Build history of the part. All positions in model axes, mm. A direction names the side the tool comes from. Round coordinates to 2 decimals unless told otherwise and drop trailing zeros. Order: outer loops, then holes, each group sorted by start corner. A loop starts at its lowest first (then second) coordinate and runs counter-clockwise, first axis right, second up. Notation, with made-up numbers: M -32.5,12.5 L -19.5,12.5 A31 cw -19.5,46.5 Z; hole C -13,67.5 d4. An arc over 180 degrees is marked long. One line per item, written item: value. Start each with the question number.
Item 1: Band-saw the part on A-A, the plane z = 0. Write the cut outline in (x, y).
Item 2: Tool access for faces 4 (the flat face through (5, 5, -7)), 5 (the flat face through (-5, 0, -6)): list every direction of +Z, -Z, +X, -X, +Y, -Y with a clear straight run to the whole face (end or side of a thin tool).
Item 3: Two-plate mould, pull along Z, no slides. Class faces 1 (the flat face through (22.5, 3, 0)), 2 (the cylindrical face through (-21.61, 3.04, 4.13)), 3 (the cylindrical face through (-1.139, 2.218, 7.514)): +Z half, -Z half, draft (parallel to the pull), parting line (faces both ways), or undercut.
Item 4: Pin check, flat tips, straight feed: pin 1 (1.5 mm diameter, centred on x = -10, y = 1, fed in from -Z); pin 2 (9 mm diameter, centred on x = 1.5, z = 4, fed in from +Y); pin 3 (1 mm diameter, centred on x = 13.5, y = 2.5, fed in from -Z). Stop position of each tip, or through.
Item 5: Band-saw the part on B-B, the plane x = 0. Write the cut outline in (y, z), then the cut area to 4 significant figures.
Item 6: Band-saw the part on C-C, the plane y = 5.5. Give the number of separate pieces and of enclosed holes in the cut face, then the cut area to 3 significant figures.
Item 7: Probe L1, parallel to X at y = 1.55, z = 0; L2, parallel to X at y = 4.8, z = 0; L3, parallel to X at y = 4.25, z = 4.5. List the from-to ranges inside material, lowest first.
```python
from build123d import *

# Parameters (mm, degrees)
SKETCH1_R           = 1.6000000000000016
BOSS_EXTRUDE1_DEPTH = 6
FILLET1_R           = 3
FILLET2_R           = 17
SKETCH2_R           = 9
CUT_EXTRUDE1_DEPTH  = 1
CHAMFER1_SIZE       = 0.5


with BuildPart() as part:
    # Sketch1 → Boss-Extrude1 (new body)
    # profile 1 of 8: a face of its own
    with BuildSketch(Plane(origin=(0, 0, 0), x_dir=(1, 0, 0), z_dir=(0, 1, 0))):
        with BuildLine():
            Line((-5.7236352085013955, -4.999999999999999), (-11.56546583584068, -5))
            ThreePointArc((-11.565465835840719, -5.000000000000114), (6.483e-14, -12.6), (11.565465835840772, -4.99999999999999))
            Line((11.565465835840783, -4.999999999999998), (5.7236352085012925, -4.999999999999999))
            ThreePointArc((5.723635208501399, -5.000000000000313), (-5.54e-14, -7.599999999999999), (-5.723635208501475, -5.0000000000002265))
        make_face()
    # profile 2 of 8: a face of its own
    with BuildSketch(Plane(origin=(0, 0, 0), x_dir=(1, 0, 0), z_dir=(0, 1, 0))):
        with BuildLine():
            Line((-11.56546583584068, 5), (-22.5, 5))
            Line((-22.5, 5), (-22.5, -5))
            Line((-22.5, -5), (-11.56546583584068, -5))
            ThreePointArc((-11.565465835840719, -5.000000000000114), (-12.6, 1.54e-15), (-11.565465835840715, 5.000000000000122))
        make_face()
        with Locations(Location((-17.499999999999996, 0, 0), (0, 0, 270))):
            Circle(SKETCH1_R, mode=Mode.SUBTRACT)
    # profile 3 of 8: a face of its own
    with BuildSketch(Plane(origin=(0, 0, 0), x_dir=(1, 0, 0), z_dir=(0, 1, 0))):
        with BuildLine():
            Line((-5.7236352085013955, 4.999999999999999), (-11.56546583584068, 5))
            ThreePointArc((-11.565465835840715, 5.000000000000122), (-12.6, 1.54e-15), (-11.565465835840719, -5.000000000000114))
            Line((-11.56546583584068, -5), (-5.7236352085013955, -4.999999999999999))
            ThreePointArc((-5.723635208501475, -5.0000000000002265), (-7.599999999999999, 9.3e-16), (-5.723635208501473, 5.000000000000228))
        make_face()
    # profile 4 of 8: a face of its own
    with BuildSketch(Plane(origin=(0, 0, 0), x_dir=(1, 0, 0), z_dir=(0, 1, 0))):
        with BuildLine():
            ThreePointArc((12.6, 0), (12.338656116684541, 2.5529522585044844), (11.56546583584077, 4.999999999999995))
            Line((11.565465835840769, 4.999999999999998), (5.723635208502053, 4.999999999999999))
            ThreePointArc((5.723635208501946, 4.9999999999996865), (7.115463006179385, 2.670240852000546), (7.599999999999999, 0))
            ThreePointArc((7.599999999999999, -1.86e-15), (7.11546300617924, -2.6702408520009326), (5.723635208501399, -5.000000000000313))
            Line((5.7236352085012925, -4.999999999999999), (11.565465835840783, -4.999999999999998))
            ThreePointArc((11.565465835840772, -4.99999999999999), (12.338656116684541, -2.552952258504483), (12.6, -3.09e-15))
        make_face()
    # profile 5 of 8: a face of its own
    with BuildSketch(Plane(origin=(0, 0, 0), x_dir=(1, 0, 0), z_dir=(0, 1, 0))):
        with BuildLine():
            ThreePointArc((11.56546583584077, 4.999999999999995), (7.072e-14, 12.6), (-11.565465835840715, 5.000000000000122))
            Line((-11.56546583584068, 5), (-5.7236352085013955, 4.999999999999999))
            ThreePointArc((-5.723635208501473, 5.000000000000228), (3.5822e-13, 7.599999999999999), (5.723635208501945, 4.999999999999687))
            Line((5.723635208502053, 4.999999999999999), (11.565465835840769, 4.999999999999998))
        make_face()
    # profile 6 of 8: a face of its own
    with BuildSketch(Plane(origin=(0, 0, 0), x_dir=(1, 0, 0), z_dir=(0, 1, 0))):
        with BuildLine():
            Line((-5.7236352085013955, 4.999999999999999), (-11.56546583584068, 5))
            ThreePointArc((-11.565465835840715, 5.000000000000122), (-12.6, 1.54e-15), (-11.565465835840719, -5.000000000000114))
            Line((-11.56546583584068, -5), (-5.7236352085013955, -4.999999999999999))
            ThreePointArc((-5.723635208501475, -5.0000000000002265), (-7.599999999999999, 9.3e-16), (-5.723635208501473, 5.000000000000228))
        make_face()
    # profile 7 of 8: a face of its own
    with BuildSketch(Plane(origin=(0, 0, 0), x_dir=(1, 0, 0), z_dir=(0, 1, 0))):
        with BuildLine():
            ThreePointArc((12.6, 0), (12.338656116684541, 2.5529522585044844), (11.56546583584077, 4.999999999999995))
            Line((11.565465835840769, 4.999999999999998), (5.723635208502053, 4.999999999999999))
            ThreePointArc((5.723635208501946, 4.9999999999996865), (7.115463006179385, 2.670240852000546), (7.599999999999999, 0))
            ThreePointArc((7.599999999999999, -1.86e-15), (7.11546300617924, -2.6702408520009326), (5.723635208501399, -5.000000000000313))
            Line((5.7236352085012925, -4.999999999999999), (11.565465835840783, -4.999999999999998))
            ThreePointArc((11.565465835840772, -4.99999999999999), (12.338656116684541, -2.552952258504483), (12.6, -3.09e-15))
        make_face()
    # profile 8 of 8: a face of its own
    with BuildSketch(Plane(origin=(0, 0, 0), x_dir=(1, 0, 0), z_dir=(0, 1, 0))):
        with BuildLine():
            Line((22.5, 4.999999999999998), (11.565465835840769, 4.999999999999998))
            ThreePointArc((11.56546583584077, 4.999999999999995), (12.338656116684541, 2.5529522585044844), (12.6, 0))
            ThreePointArc((12.6, -3.09e-15), (12.338656116684541, -2.552952258504483), (11.565465835840772, -4.99999999999999))
            Line((11.565465835840783, -4.999999999999998), (22.5, -4.999999999999998))
            Line((22.5, -4.999999999999998), (22.5, 4.999999999999998))
        make_face()
        with Locations(Location((17.499999999999996, 0, 0), (0, 0, 270))):
            Circle(SKETCH1_R, mode=Mode.SUBTRACT)
    extrude(amount=BOSS_EXTRUDE1_DEPTH)

    # Fillet1
    fillet1_edges = [part.edges().sort_by_distance(p)[0] for p in [
        (22.5, 3, -4.999999999999998),
        (22.5, 3, 4.999999999999998),
        (-22.5, 3, 5),
        (-22.5, 3, -5),
    ]]
    fillet(fillet1_edges, radius=FILLET1_R)

    # Fillet2
    fillet2_edges = [part.edges().sort_by_distance(p)[0] for p in [
        (11.56546583584077, 3, -4.9999999999999964),
        (-11.5654658358407, 3, -5.00000000000006),
        (11.565465835840776, 3, 4.999999999999994),
        (-11.5654658358407, 3, 5.000000000000057),
    ]]
    fillet(fillet2_edges, radius=FILLET2_R)

    # Sketch2 → Cut-Extrude1 (cut)
    with BuildSketch(Plane(origin=(0, 6, 0), x_dir=(1, 0, 0), z_dir=(0, 1, 0))):
        with Locations(Location((0, 0, 0), (0, 0, 270))):
            Circle(SKETCH2_R)
    extrude(amount=-CUT_EXTRUDE1_DEPTH, mode=Mode.SUBTRACT)

    # Chamfer1
    chamfer1_edges = [part.edges().sort_by_distance(p)[0] for p in [
        (-5.7236352085019595, 5, 4.999999999999671),
    ]]
    chamfer(chamfer1_edges, length=CHAMFER1_SIZE)


solid = part.part
```
Output:
1. outline: M -22.5,0 L -19.1,0 L -19.1,6 L -22.5,6 Z; M -15.9,0 L -7.6,0 L -7.6,4.5 L -8.1,5 L -9,5 L -9,6 L -15.9,6 Z; M 7.6,0 L 15.9,0 L 15.9,6 L 9,6 L 9,5 L 8.1,5 L 7.6,4.5 Z; M 19.1,0 L 22.5,0 L 22.5,6 L 19.1,6 Z
2. face 4: +Y
2. face 5: +Z, -Z, +X, -X, -Y
3. face 1: draft
3. face 2: +Z half
3. face 3: undercut
4. pin 1: stops at z = -8.67
4. pin 2: stops at y = 5
4. pin 3: stops at z = -6.42
5. outline: M 0,-12.6 L 6,-12.6 L 6,-9 L 5,-9 L 5,-8.1 L 4.5,-7.6 L 0,-7.6 Z; M 0,7.6 L 4.5,7.6 L 5,8.1 L 5,9 L 6,9 L 6,12.6 L 0,12.6 Z
5. area: 56.95 mm²
6. separate pieces: 1
6. enclosed holes: 3
6. area: 456 mm²
7. L1: x = -22.5 to -19.1, -15.9 to -7.6, 7.6 to 15.9, 19.1 to 22.5
7. L2: x = -22.5 to -19.1, -15.9 to -7.9, 7.9 to 15.9, 19.1 to 22.5
7. L3: x = -21.16 to -6.12, 6.12 to 21.16
